Geometry check sheet. Reference: the model listing, model coordinates, mm. A direction names the side the tool comes from. Round coordinates to 2 decimals unless told otherwise and drop trailing zeros. Loops run counter-clockwise (first coordinate to the right, second up) from the corner with the lowest first, then second, coordinate; pieces in that order, holes last. Notation, with made-up numbers: (-26, -13.5) - (16, -13.5) arc R34 cw to (16, 16.5) - close; hole circle Ø1 at (16.25, 79.5). An arc over 180 degrees is marked (long way). Answer in a Markdown table with one row per item. Add a question column.
```python
from build123d import *

# Parameters (mm, degrees)
BASPROSKE_W     = 17.5
BASPROSKE_H     = 6
TOOTHCUT_DEPTH  = 20.448650339
TEETHCUTS_COUNT = 10
TEETHCUTS_ANGLE = 324
BORSKE_R        = 2.35
BORE_DEPTH      = 50.0000508
SCALE_1_SCALE   = 1.065


with BuildPart() as part:
    # BasProSke → Base-Revolve (revolve)
    with BuildSketch(Plane(origin=(0, 0, 0), x_dir=(1, 0, 0), z_dir=(0, 1, 0)), mode=Mode.PRIVATE) as base_revolve_sk:
        with Locations((8.75, 3)):
            Rectangle(BASPROSKE_W, BASPROSKE_H)
    revolve(base_revolve_sk.sketch.rotate(Axis((-10, 0, 0), (1, 0, 0)), 180), axis=Axis((-10, 0, 0), (1, 0, 0)))

    # TooCutSke → ToothCut (cut, through all)
    with BuildSketch(Plane(origin=(0, 0, 0), x_dir=(0, 0, -1), z_dir=(1, 0, 0))):
        with BuildLine():
            ThreePointArc((0.59278292, 3.701838653), (0, 3.749), (-0.59278292, 3.701838653))
            ThreePointArc((-0.59278292, 3.701838653), (-0.846593509, 4.924114224), (-1.775771316, 5.757784417))
            ThreePointArc((-1.775771316, 5.757784417), (0, 6.0254), (1.775771316, 5.757784417))
            ThreePointArc((1.775771316, 5.757784417), (0.846593509, 4.924114224), (0.59278292, 3.701838653))
        make_face()
    toothcut = extrude(amount=TOOTHCUT_DEPTH, mode=Mode.SUBTRACT)

    # TeethCuts: ToothCut ×10 about axis
    teethcuts_axis = Axis((-10, 0, 0), (1, 0, 0))
    for i in range(1, TEETHCUTS_COUNT):
        add(toothcut.rotate(teethcuts_axis, i * TEETHCUTS_ANGLE / (TEETHCUTS_COUNT - 1)), mode=Mode.SUBTRACT)

    # BorSke → Bore (cut, symmetric)
    with BuildSketch(Plane(origin=(0, 0, 0), x_dir=(0, 0, -1), z_dir=(1, 0, 0))):
        with Locations(Location((0, 0, 0), (0, 0, 180))):
            Circle(BORSKE_R)
    extrude(amount=BORE_DEPTH, both=True, mode=Mode.SUBTRACT)


with BuildPart() as part_1:
    # Масштаб1: scaled about (8.75, 0, 0)
    add(part.part.scale(SCALE_1_SCALE).moved(Location((-0.56875, 0, 0))))

    # Эскиз2 → Повернуть1 (revolve)
    with BuildSketch(Plane(origin=(0, 0, 0), x_dir=(1, 0, 0), z_dir=(0, 1, 0))):
        Polygon((-0.56875, 3.5), (-0.56875, 6.39), (-1.76875, 6.39), (-1.76875, 5), (-2.96875, 5), (-2.96875, 3.924264069), (-2.544485931, 3.5), align=None)
    revolve(axis=Axis((0, 0, 0), (-1, 0, 0)))


solid = part_1.part
```
Q1. Scan lines: line 1 (Y direction, x = -1.85, z = 0); line 2 (Y direction, x = -1.5, z = 0); line 3 (Y direction, x = 11.75, z = -4.25). Record each from-to range of solid material in increasing order. Write a range as from..to.
Q2. Cross-section at D-D, the plane z = 4.25. Enter the section's corners in (x, y), plus the area to 3 significant figures.
Q3. Set-up check for faces 1 (the cylindrical face through (8.88, -1.691, -1.845)), 2 (the flat face through (-0.569, 4, 3)), 3 (the cylindrical face through (-1.543, 1.341, -3.233)): record each of +Z, -Z, +X, -X, +Y, -Y from which the full face is reachable in a straight line by a thin tool's end or side.
Q4. Cross-section at A-A, the plane z = 0. Enter the section's corners in (x, y).
Q5. Depth check by flat-ended pin: P1, Ø4, axis at y = 1.5, z = -1, coming from the -X side; P2, Ø1.5, axis at x = 6.5, y = 5, coming from the +Z side (3 decimals); P3, Ø4, axis at x = 14, z = -3.5, coming from the +Y side. Enter the tip coordinate at first touch or a pass-through.
Q6. Cross-section at C-C, the plane y = 4.5. Enter the section's corners in (x, z), plus the area to 3 significant figures.
Q7. Cross-section at B-B, the plane x = -1. Enter the section's corners in (y, z), plus the area to 3 significant figures.
Q8. Release check for a two-part mould opening along Y. For faces 4 (the cylindrical face through (8.62, -1.242, -3.795)), 5 (the cylindrical face through (8.62, 4.73, -2.35)), 6 (the cylindrical face through (-2.38, 4.88, 1.08)) record: +Y half, -Y half, draft (parallel to the pull), parting line (faces both ways), or undercut.
Check sheet entries:
| question | item | result |
|---|---|---|
| 1 | line 1 | -5..-3.5, 3.5..5 |
| 1 | line 2 | -6.39..-3.5, 3.5..6.39 |
| 1 | line 3 | -3.85..-2.1, -0.73..0.73, 2.1..3.85 |
| 2 | outline | (-2.97, -2.63) - (-1.77, -2.63) - (-1.77, -4.77) - (-0.57, -4.77) - (-0.57, -3.85) - (18.07, -3.85) - (18.07, -2.1) - (-0.57, -2.1) - (-0.57, -0.73) - (18.07, -0.73) - (18.07, 0.73) - (-0.57, 0.73) - (-0.57, 2.1) - (18.07, 2.1) - (18.07, 3.85) - (-0.57, 3.85) - (-0.57, 4.77) - (-1.77, 4.77) - (-1.77, 2.63) - (-2.97, 2.63) - close |
| 2 | area | 111 mm² |
| 3 | face 1 | +X, -X |
| 3 | face 2 | +X |
| 3 | face 3 | -X |
| 4 | outline | (-2.97, -5) - (-1.77, -5) - (-1.77, -6.39) - (-0.57, -6.39) - (-0.57, -3.99) - (18.07, -3.99) - (18.07, -2.5) - (-0.57, -2.5) - (-0.57, -3.5) - (-2.54, -3.5) - (-2.97, -3.92) - close; (-2.97, 3.92) - (-2.54, 3.5) - (-0.57, 3.5) - (-0.57, 2.5) - (18.07, 2.5) - (18.07, 3.99) - (-0.57, 3.99) - (-0.57, 6.39) - (-1.77, 6.39) - (-1.77, 5) - (-2.97, 5) - close |
| 5 | P1 | x = -2.85 |
| 5 | P2 | z = 2.365 |
| 5 | P3 | y = 6.12 |
| 6 | outline | (-2.97, -2.18) - (-1.77, -2.18) - (-1.77, -4.54) - (-0.57, -4.54) - (-0.57, -2.31) - (18.07, -2.31) - (18.07, -0.64) - (-0.57, -0.64) - (-0.57, 0.64) - (18.07, 0.64) - (18.07, 2.31) - (-0.57, 2.31) - (-0.57, 4.54) - (-1.77, 4.54) - (-1.77, 2.18) - (-2.97, 2.18) - close |
| 6 | area | 78.2 mm² |
| 7 | outline | circle Ø12.78 at (0, 0); hole circle Ø7 at (0, 0) |
| 7 | area | 89.8 mm² |
| 8 | face 4 | undercut |
| 8 | face 5 | undercut |
| 8 | face 6 | parting line |
